Work out the finished part from the listing and answer in its coordinate system (mm). A direction names the side the tool comes from. Give positions to 0.01 mm unless a question says otherwise; leave off trailing zeros. Write each loop counter-clockwise with the first axis right and the second up, starting at its lowest first coordinate (ties: lowest second). Pieces come first, ordered by that corner, then holes.
1) Find section D-D (z = -35.5). Determine the outline of the cut face in (x, y), plus the area to 3 significant figures.
2) Determine the mould class of faces 5 (the face through (1, -15, -47)), 6 (the face through (1, 20, 45.5)), 7 (the face through (1, 5, 0)) for opening direction Y: pulls with the +Y half, pulls with the -Y half, needs draft (parallel to the pull), parting line crosses it, or undercut.
3) Find section A-A (z = -13.5). Determine the outline of the cut face in (x, y), plus the area to 3 significant figures.
4) Straight lines are drawn through the part: probe 1 along Z at (x, y) = (1.35, -0.5); probe 2 along Y at (x, z) = (1.4, 11); probe 3 along Y at (x, z) = (2.9, 2). For each, find the intervals that lie inside material, in ascending order.
5) Find section C-C (y = -16.5). Determine the outline of the cut face in (x, z).
6) Find section B-B (z = 1.5). Determine the outline of the cut face in (x, y).
7) Given pin 1 Ø1.5 at (x, z) = (1, 8.5) entering from -Y; pin 2 Ø0.9 at (x, y) = (1, -24) entering from +Z; pin 3 Ø0.9 at (x, y) = (1, -23) entering from -Z; pin 4 Ø4 at (y, z) = (-18.5, -2.5) entering from -X, each flat-ended and moving along its own axis, determine where each tip first touches the part or whether it passes through.
8) A tool of negligible diameter and unlimited length cuts with its end or side. For faces 1 (the face through (1, -24, -37.722)), 2 (the face through (1, 0, -20)), 3 (the face through (1, -20, -45.5)), 4 (the face through (1, 22, -32)), from which of +Z, -Z, +X, -X, +Y, -Y can it reach the whole face along a straight path? Write none if from no direction.
```python
from build123d import *

# Parameters (mm, degrees)
ESBO_O1_W                = 97
ESBO_O1_H                = 50
RESSALTO_EXTRUS_O1_DEPTH = 3
CORTE_EXTRUS_O1_REACH    = 56.647
ESBO_O2_W                = 10.782222222
ESBO_O2_H                = 3
CORTE_EXTRUS_O2_REACH    = 56.647
ESBO_O4_W                = 3
ESBO_O4_H                = 10
CORTE_EXTRUS_O5_REACH    = 56.647
ESBO_O3_W                = 40
ESBO_O3_H                = 10


with BuildPart() as part:
    # Esboço1 → Ressalto-extrusão1 (new body)
    with BuildSketch(Plane(origin=(0, 0, 0), x_dir=(0, 0, -1), z_dir=(1, 0, 0))):
        Rectangle(ESBO_O1_W, ESBO_O1_H)
    extrude(amount=RESSALTO_EXTRUS_O1_DEPTH)

    # Esboço2 → Corte-extrusão1 (cut, up to next)
    with BuildSketch(Plane.ZY, mode=Mode.PRIVATE) as corte_extrus_o1_sk1:
        with Locations((-10.771111111, 23.5)):
            Rectangle(ESBO_O2_W, ESBO_O2_H)
    corte_extrus_o1_tool1 = extrude(corte_extrus_o1_sk1.sketch, amount=-CORTE_EXTRUS_O1_REACH, mode=Mode.PRIVATE) & part.part
    # Esboço2 → Corte-extrusão1 (cut, up to next)
    with BuildSketch(Plane.ZY, mode=Mode.PRIVATE) as corte_extrus_o1_sk2:
        with Locations((-32.331111111, 23.5)):
            Rectangle(ESBO_O2_W, ESBO_O2_H)
    corte_extrus_o1_tool2 = extrude(corte_extrus_o1_sk2.sketch, amount=-CORTE_EXTRUS_O1_REACH, mode=Mode.PRIVATE) & part.part
    # Esboço2 → Corte-extrusão1 (cut, up to next)
    with BuildSketch(Plane.ZY, mode=Mode.PRIVATE) as corte_extrus_o1_sk3:
        with Locations((10.788888889, 23.5)):
            Rectangle(ESBO_O2_W, ESBO_O2_H)
    corte_extrus_o1_tool3 = extrude(corte_extrus_o1_sk3.sketch, amount=-CORTE_EXTRUS_O1_REACH, mode=Mode.PRIVATE) & part.part
    # Esboço2 → Corte-extrusão1 (cut, up to next)
    with BuildSketch(Plane.ZY, mode=Mode.PRIVATE) as corte_extrus_o1_sk4:
        with Locations((32.348888889, 23.5)):
            Rectangle(ESBO_O2_W, ESBO_O2_H)
    corte_extrus_o1_tool4 = extrude(corte_extrus_o1_sk4.sketch, amount=-CORTE_EXTRUS_O1_REACH, mode=Mode.PRIVATE) & part.part
    # Esboço2 → Corte-extrusão1 (cut, up to next)
    with BuildSketch(Plane.ZY, mode=Mode.PRIVATE) as corte_extrus_o1_sk5:
        with Locations((-32.331111111, -23.5)):
            Rectangle(ESBO_O2_W, ESBO_O2_H)
    corte_extrus_o1_tool5 = extrude(corte_extrus_o1_sk5.sketch, amount=-CORTE_EXTRUS_O1_REACH, mode=Mode.PRIVATE) & part.part
    # Esboço2 → Corte-extrusão1 (cut, up to next)
    with BuildSketch(Plane.ZY, mode=Mode.PRIVATE) as corte_extrus_o1_sk6:
        with Locations((32.348888889, -23.5)):
            Rectangle(ESBO_O2_W, ESBO_O2_H)
    corte_extrus_o1_tool6 = extrude(corte_extrus_o1_sk6.sketch, amount=-CORTE_EXTRUS_O1_REACH, mode=Mode.PRIVATE) & part.part
    # Esboço2 → Corte-extrusão1 (cut, up to next)
    with BuildSketch(Plane.ZY, mode=Mode.PRIVATE) as corte_extrus_o1_sk7:
        with Locations((-10.771111111, -23.5)):
            Rectangle(ESBO_O2_W, ESBO_O2_H)
    corte_extrus_o1_tool7 = extrude(corte_extrus_o1_sk7.sketch, amount=-CORTE_EXTRUS_O1_REACH, mode=Mode.PRIVATE) & part.part
    # Esboço2 → Corte-extrusão1 (cut, up to next)
    with BuildSketch(Plane.ZY, mode=Mode.PRIVATE) as corte_extrus_o1_sk8:
        with Locations((10.788888889, -23.5)):
            Rectangle(ESBO_O2_W, ESBO_O2_H)
    corte_extrus_o1_tool8 = extrude(corte_extrus_o1_sk8.sketch, amount=-CORTE_EXTRUS_O1_REACH, mode=Mode.PRIVATE) & part.part
    add(corte_extrus_o1_tool1.solids().sort_by_distance((0, 23.5, -10.771111))[0], mode=Mode.SUBTRACT)
    add(corte_extrus_o1_tool2.solids().sort_by_distance((0, 23.5, -32.331111))[0], mode=Mode.SUBTRACT)
    add(corte_extrus_o1_tool3.solids().sort_by_distance((0, 23.5, 10.788889))[0], mode=Mode.SUBTRACT)
    add(corte_extrus_o1_tool4.solids().sort_by_distance((0, 23.5, 32.348889))[0], mode=Mode.SUBTRACT)
    add(corte_extrus_o1_tool5.solids().sort_by_distance((0, -23.5, -32.331111))[0], mode=Mode.SUBTRACT)
    add(corte_extrus_o1_tool6.solids().sort_by_distance((0, -23.5, 32.348889))[0], mode=Mode.SUBTRACT)
    add(corte_extrus_o1_tool7.solids().sort_by_distance((0, -23.5, -10.771111))[0], mode=Mode.SUBTRACT)
    add(corte_extrus_o1_tool8.solids().sort_by_distance((0, -23.5, 10.788889))[0], mode=Mode.SUBTRACT)

    # Esboço4 → Corte-extrusão2 (cut, up to next)
    with BuildSketch(Plane.ZY, mode=Mode.PRIVATE) as corte_extrus_o2_sk1:
        with Locations((47, 20)):
            Rectangle(ESBO_O4_W, ESBO_O4_H)
    corte_extrus_o2_tool1 = extrude(corte_extrus_o2_sk1.sketch, amount=-CORTE_EXTRUS_O2_REACH, mode=Mode.PRIVATE) & part.part
    # Esboço4 → Corte-extrusão2 (cut, up to next)
    with BuildSketch(Plane.ZY, mode=Mode.PRIVATE) as corte_extrus_o2_sk2:
        with Locations((-47, -20)):
            Rectangle(ESBO_O4_W, ESBO_O4_H)
    corte_extrus_o2_tool2 = extrude(corte_extrus_o2_sk2.sketch, amount=-CORTE_EXTRUS_O2_REACH, mode=Mode.PRIVATE) & part.part
    # Esboço4 → Corte-extrusão2 (cut, up to next)
    with BuildSketch(Plane.ZY, mode=Mode.PRIVATE) as corte_extrus_o2_sk3:
        with Locations((-47, 20)):
            Rectangle(ESBO_O4_W, ESBO_O4_H)
    corte_extrus_o2_tool3 = extrude(corte_extrus_o2_sk3.sketch, amount=-CORTE_EXTRUS_O2_REACH, mode=Mode.PRIVATE) & part.part
    # Esboço4 → Corte-extrusão2 (cut, up to next)
    with BuildSketch(Plane.ZY, mode=Mode.PRIVATE) as corte_extrus_o2_sk4:
        with Locations((47, -20)):
            Rectangle(ESBO_O4_W, ESBO_O4_H)
    corte_extrus_o2_tool4 = extrude(corte_extrus_o2_sk4.sketch, amount=-CORTE_EXTRUS_O2_REACH, mode=Mode.PRIVATE) & part.part
    # Esboço4 → Corte-extrusão2 (cut, up to next)
    with BuildSketch(Plane.ZY, mode=Mode.PRIVATE) as corte_extrus_o2_sk5:
        with Locations((47, 0)):
            Rectangle(ESBO_O4_W, ESBO_O4_H)
    corte_extrus_o2_tool5 = extrude(corte_extrus_o2_sk5.sketch, amount=-CORTE_EXTRUS_O2_REACH, mode=Mode.PRIVATE) & part.part
    # Esboço4 → Corte-extrusão2 (cut, up to next)
    with BuildSketch(Plane.ZY, mode=Mode.PRIVATE) as corte_extrus_o2_sk6:
        with Locations((-47, 0)):
            Rectangle(ESBO_O4_W, ESBO_O4_H)
    corte_extrus_o2_tool6 = extrude(corte_extrus_o2_sk6.sketch, amount=-CORTE_EXTRUS_O2_REACH, mode=Mode.PRIVATE) & part.part
    add(corte_extrus_o2_tool1.solids().sort_by_distance((0, 20, 47))[0], mode=Mode.SUBTRACT)
    add(corte_extrus_o2_tool2.solids().sort_by_distance((0, -20, -47))[0], mode=Mode.SUBTRACT)
    add(corte_extrus_o2_tool3.solids().sort_by_distance((0, 20, -47))[0], mode=Mode.SUBTRACT)
    add(corte_extrus_o2_tool4.solids().sort_by_distance((0, -20, 47))[0], mode=Mode.SUBTRACT)
    add(corte_extrus_o2_tool5.solids().sort_by_distance((0, 0, 47))[0], mode=Mode.SUBTRACT)
    add(corte_extrus_o2_tool6.solids().sort_by_distance((0, 0, -47))[0], mode=Mode.SUBTRACT)

    # Esboço3 → Corte-extrusão5 (cut, up to next)
    with BuildSketch(Plane(origin=(0, 0, 0), x_dir=(0, 0, -1), z_dir=(1, 0, 0)), mode=Mode.PRIVATE) as corte_extrus_o5_sk1:
        Rectangle(ESBO_O3_W, ESBO_O3_H)
    corte_extrus_o5_tool1 = extrude(corte_extrus_o5_sk1.sketch, amount=CORTE_EXTRUS_O5_REACH, mode=Mode.PRIVATE) & part.part
    add(corte_extrus_o5_tool1.solids().sort_by_distance((0, 0, 0))[0], mode=Mode.SUBTRACT)


solid = part.part
```
Results:
1. outline: (0, -22) - (3, -22) - (3, 22) - (0, 22) - close
1. area: 132 mm2
2. face 5: pulls with the -Y half
2. face 6: needs draft
2. face 7: undercut
3. outline: (0, -22) - (3, -22) - (3, -5) - (0, -5) - close; (0, 5) - (3, 5) - (3, 22) - (0, 22) - close
3. area: 102 mm2
4. probe 1: z = -45.5 to -20, 20 to 45.5
4. probe 2: y = -22 to -5, 5 to 22
4. probe 3: y = -25 to -5, 5 to 25
5. outline: (0, -45.5) - (3, -45.5) - (3, 45.5) - (0, 45.5) - close
6. outline: (0, -25) - (3, -25) - (3, -5) - (0, -5) - close; (0, 5) - (3, 5) - (3, 25) - (0, 25) - close
7. pin 1: stops at y = -22
7. pin 2: stops at z = 45.5
7. pin 3: stops at z = -45.5
7. pin 4: stops at x = 0
8. face 1: +X, -X, -Y
8. face 2: +X, -X
8. face 3: -Z, +X, -X, -Y
8. face 4: +X, -X, +Y
